Geometry: final body of the model. Coordinates: model frame, mm. Face numbers are marked on the shaded views. A direction names the side the tool comes from. Give positions to 0.01 mm unless a question says otherwise; leave off trailing zeros. Loops run counter-clockwise (first coordinate to the right, second up) from the corner with the lowest first, then second, coordinate; pieces in that order, holes last. Notation, with made-up numbers: M 72,40.5 L 102,40.5 A29 ccw 102,72.5 Z; hole C -1,73 d4. An arc over 180 degrees is marked long. Put each result on its own line as item: value.
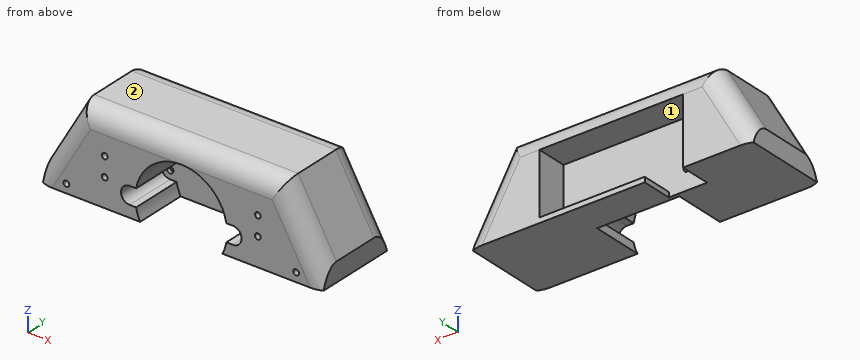
```python
from build123d import *

# Parameters (mm, degrees)
BOSS_EXTRUDE2_DEPTH = 45
FILLET2_R           = 10
FILLET3_R           = 10
SKETCH6_R           = 1.5
CUT_EXTRUDE5_DEPTH  = 10
SKETCH7_R           = 1.5
CUT_EXTRUDE6_DEPTH  = 10
CUT_EXTRUDE7_DEPTH  = 27
SKETCH3_W           = 75
SKETCH3_H           = 32
CUT_EXTRUDE8_DEPTH  = 16
SKETCH11_R          = 1.75
CUT_EXTRUDE9_DEPTH  = 20
SKETCH12_W          = 20
SKETCH12_H          = 2.641016152
CUT_EXTRUDE11_DEPTH = 16


with BuildPart() as part:
    # Sketch2 → Boss-Extrude2 (new body)
    with BuildSketch(Plane(origin=(0, 0, 0), x_dir=(1, 0, 0), z_dir=(0, 1, 0))):
        Polygon((-73.275, 22.320508076), (73.275, 22.320508076), (73.275, 12.320508076), (53.275, -22.320508076), (-53.275, -22.320508076), (-73.275, 12.320508076), align=None)
    extrude(amount=BOSS_EXTRUDE2_DEPTH)

    # Fillet2
    fillet2_edges = [part.edges().sort_by_distance(p)[0] for p in [
        (63.275, 45, 5),
        (0, 45, 22.320508076),
        (-63.275, 45, 5),
    ]]
    fillet(fillet2_edges, radius=FILLET2_R)

    # Fillet3
    fillet3_edges = [part.edges().sort_by_distance(p)[0] for p in [
        (-63.275, 0, 5),
        (63.275, 0, 5),
        (0, 0, 22.320508076),
    ]]
    fillet(fillet3_edges, radius=FILLET3_R)

    # Sketch6 → Cut-Extrude5 (cut)
    with BuildSketch(Plane(origin=(0, 0, 0), x_dir=(-1, 0, 0), z_dir=(0, -1, 0))):
        with Locations(Location((40, -2.320508076, 0), (0, 0, 90))):
            Circle(SKETCH6_R)
        with Locations(Location((-40, -2.320508076, 0), (0, 0, 270))):
            Circle(SKETCH6_R)
        with Locations(Location((60, 17.679491924, 0), (0, 0, 90))):
            Circle(SKETCH6_R)
        with Locations(Location((-60, 17.679491924, 0), (0, 0, 270))):
            Circle(SKETCH6_R)
    extrude(amount=-CUT_EXTRUDE5_DEPTH, mode=Mode.SUBTRACT)

    # Sketch7 → Cut-Extrude6 (cut)
    with BuildSketch(Plane(origin=(0, 0, 0), x_dir=(-1, 0, 0), z_dir=(0, -1, 0))):
        with Locations(Location((40, 7.679491924, 0), (0, 0, 90))):
            Circle(SKETCH7_R)
        with Locations(Location((-40, 7.679491924, 0), (0, 0, 270))):
            Circle(SKETCH7_R)
    extrude(amount=-CUT_EXTRUDE6_DEPTH, mode=Mode.SUBTRACT)

    # Sketch9 → Cut-Extrude7 (cut)
    with BuildSketch(Plane(origin=(0, 0, 0), x_dir=(-1, 0, 0), z_dir=(0, -1, 0))):
        with BuildLine():
            Line((27, 7.179491924), (23.574350468, 7.179491924))
            ThreePointArc((23.574350468, 7.179491924), (0, -12.320508076), (-23.574350468, 7.179491924))
            Line((-23.574350468, 7.179491924), (-27, 7.179491924))
            ThreePointArc((-27, 7.179491924), (-31.5, 11.679491924), (-27, 16.179491924))
            Line((-27, 16.179491924), (-23.574350468, 16.179491924))
            ThreePointArc((-23.574350468, 16.179491924), (0, 35.679491924), (23.574350468, 16.179491924))
            Line((23.574350468, 16.179491924), (27, 16.179491924))
            ThreePointArc((27, 16.179491924), (31.5, 11.679491924), (27, 7.179491924))
        make_face()
    extrude(amount=-CUT_EXTRUDE7_DEPTH, mode=Mode.SUBTRACT)

    # Sketch3 → Cut-Extrude8 (cut)
    with BuildSketch(Plane(origin=(0, 45, 0), x_dir=(1, 0, 0), z_dir=(0, 1, 0))):
        with Locations((0, 3.679491924)):
            Rectangle(SKETCH3_W, SKETCH3_H)
    extrude(amount=-CUT_EXTRUDE8_DEPTH, mode=Mode.SUBTRACT)

    # Sketch11 → Cut-Extrude9 (cut)
    with BuildSketch(Plane(origin=(0, 29, 0), x_dir=(1, 0, 0), z_dir=(0, 1, 0))):
        with Locations(Location((27, 11.679491924, 0), (0, 0, 270))):
            Circle(SKETCH11_R)
        with Locations(Location((-27, 11.679491924, 0), (0, 0, 90))):
            Circle(SKETCH11_R)
    extrude(amount=-CUT_EXTRUDE9_DEPTH, mode=Mode.SUBTRACT)

    # Sketch12 → Cut-Extrude11 (cut)
    with BuildSketch(Plane(origin=(0, 45, 0), x_dir=(1, 0, 0), z_dir=(0, 1, 0))):
        with Locations((-27.5, 21)):
            Rectangle(SKETCH12_W, SKETCH12_H)
    extrude(amount=-CUT_EXTRUDE11_DEPTH, mode=Mode.SUBTRACT)


solid = part.part
```
Item 1: Section A-A on x = -33. Output: boundary loops of the cut face in (y, z), then the cut area to 3 significant figures.
Output values:
outline: M 0,-22.32 L 29,-22.32 L 29,12.32 L 45,12.32 A10 ccw 35,22.32 L 10,22.32 A10 ccw 0,12.32 Z
area: 1,410 mm²
Item 2: Line query: probe 1 along Z at (x, y) = (40, 7); probe 2 along Z at (x, y) = (39, 4); probe 3 along X at (y, z) = (33, -16) (3 decimals). Output: solid intervals per line, ascending. Write a range as [from, to].
Output values:
probe 1: [-22.32, -9.18], [-6.18, 0.82], [3.82, 21.86]
probe 2: [-22.32, -8.8], [-6.56, 1.2], [3.44, 20.32]
probe 3: [-73.275, -37.5], [37.5, 73.275]
Item 3: Pin query (flat end, axial travel): pin 1 Ø5 at (y, z) = (34, -5.5) entering from -X; pin 2 Ø2.5 at (x, z) = (60.5, -18.5) entering from -Y; pin 3 Ø1 at (x, y) = (8, 8.5) entering from -Z; pin 4 Ø3 at (x, z) = (-27, -11.68) entering from -Y. Return the tip coordinate at first contact, or that it passes through.
Output values:
pin 1: x = -70.78
pin 2: y = 0
pin 3: z = 10.76
pin 4: through
Item 4: Set-up query: the marked faces 1 and 2. Return all of +Z, -Z, +X, -X, +Y, -Y with unobstructed straight access to the full face (end or side cutting, diameter ignored); none if empty.
Output values:
face 1: +Y
face 2: +Z, +X, -X, +Y, -Y
Item 5: Section D-D on x = -1.5. Output: boundary loops of the cut face in (y, z), then the cut area to 3 significant figures.
Output values:
outline: M 0,12.27 L 27,12.27 L 27,-22.32 L 45,-22.32 L 45,-19.68 L 29,-19.68 L 29,12.32 L 45,12.32 A10 ccw 35,22.32 L 10,22.32 A10 ccw 0,12.32 Z
area: 520 mm²
Item 6: Section B-B on y = 25. Output: boundary loops of the cut face in (x, z) (1 decimal), then the cut area to 3 significant figures.
Output values:
outline: M -73.3,-22.3 L -21.5,-22.3 A24 cw -23.6,-16.2 L -27,-16.2 A4.5 cw -27,-7.2 L -23.6,-7.2 A24 cw 23.6,-7.2 L 27,-7.2 A4.5 cw 27,-16.2 L 23.6,-16.2 A24 cw 21.5,-22.3 L 73.3,-22.3 L 73.3,-12.3 L 53.3,22.3 L -53.3,22.3 L -73.3,-12.3 Z
area: 4,330 mm²
Item 7: Section C-C on x = 17.5. Output: boundary loops of the cut face in (y, z).
Output values:
outline: M 0,4.74 L 27,4.74 L 27,-22.32 L 45,-22.32 L 45,-19.68 L 29,-19.68 L 29,12.32 L 45,12.32 A10 ccw 35,22.32 L 10,22.32 A10 ccw 0,12.32 Z
